from build123d import *

# Parameters (mm, degrees)
BOSS_EXTRUDE1_DEPTH = 3
SKETCH2_W           = 3.5
SKETCH2_H           = 35
CUT_EXTRUDE7_DEPTH  = 3
FILLET5_R           = 1.5


with BuildPart() as part:
    # Sketch1 → Boss-Extrude1 (new body)
    with BuildSketch(Plane.XY):
        Polygon((68.5, 46), (-68.5, 46), (-68.5, 42.5), (-72, 42.5), (-72, 3.5), (-68.5, 3.5), (-68.5, 0), (68.5, 0), (68.5, 3.5), (72, 3.5), (72, 42.5), (68.5, 42.5), align=None)
    extrude(amount=BOSS_EXTRUDE1_DEPTH)

    # Sketch2 → Cut-Extrude7 (cut)
    with BuildSketch(Plane.XY.offset(3)):
        with Locations((-68.25, 23)):
            Rectangle(SKETCH2_W, SKETCH2_H)
        with Locations((68.25, 23)):
            Rectangle(SKETCH2_W, SKETCH2_H)
    extrude(amount=-CUT_EXTRUDE7_DEPTH, mode=Mode.SUBTRACT)

    # Fillet5
    fillet5_edges = [part.edges().sort_by_distance(p)[0] for p in [
        (-70, 5.5, 1.5),
        (-70, 40.5, 1.5),
        (-66.5, 40.5, 1.5),
        (-66.5, 5.5, 1.5),
        (70, 40.5, 1.5),
        (70, 5.5, 1.5),
        (66.5, 5.5, 1.5),
        (66.5, 40.5, 1.5),
    ]]
    fillet(fillet5_edges, radius=FILLET5_R)


solid = part.part
The model under review builds one solid part; all positions refer to its coordinate system, in mm. A direction names the side the tool comes from. Coordinates: 2 decimals unless noted, no trailing zeros. Loops run counter-clockwise (first coordinate to the right, second up) from the corner with the lowest first, then second, coordinate; pieces in that order, holes last. Notation, with made-up numbers: M 10.25,-12.75 L 59.25,-12.75 A33 ccw 59.25,26.25 Z; hole C 27.25,78.25 d5. An arc over 180 degrees is marked long. Put each result on its own line as item: value. Start each with the question number.
Q1. Add section B-B (z = 2.15). Write out the cut boundary in (x, y), and give its area (3 significant figures).
Q2. For faces 5 (the flat face through (-68.5, 44, 1)), 6 (the flat face through (1, 46, 1)), 7 (the flat face through (68.5, 44, 1)), 8 (the flat face through (-70, 3.5, 1)), 9 (the flat face through (66.5, 23, 2)), list the 3-axis set-ups (+Z, -Z, +X, -X, +Y, -Y) from which the entire face can be reached by the end or side of a thin tool; tool diameter is ignored.
Q3. Add section A-A (y = 13). Write out the cut boundary in (x, z), and give its area (3 significant figures).
Q4. Wall thickness on line 1 (X direction, y = 22, z = 0.45); line 2 (X direction, y = 39.5, z = 2.15); line 3 (X direction, y = 43.5, z = 2.3): over which ranges is each line inside the solid? List them lowest first.
Q5. The part is to be moulded in two halves that separate along Y. For faces 1 (the flat face through (70, 42.5, 1)), 2 (the flat face through (-66.5, 23, 2)), 3 (the flat face through (70, 3.5, 1)), 4 (the flat face through (68.5, 2, 1)), say which applies: +Y half, -Y half, draft (parallel to the pull), parting line (faces both ways), or undercut.
Q6. Clearance check with flat-ended pins moving along their axes: pin 1 (1.5 mm diameter, centred on x = -71, z = 1, fed in from +Y); pin 2 (1.5 mm diameter, centred on x = 70.5, z = 1, fed in from -Y); pin 3 (1.5 mm diameter, centred on y = 44, z = 1.5, fed in from +X). State where each tip first meets the part, or that it passes through.
Answers:
1. outline: M -72,3.5 L -68.5,3.5 L -68.5,0 L 68.5,0 L 68.5,3.5 L 72,3.5 L 72,42.5 L 68.5,42.5 L 68.5,46 L -68.5,46 L -68.5,42.5 L -72,42.5 Z; hole M -70,7 A1.5 ccw -68.5,5.5 L -68,5.5 A1.5 ccw -66.5,7 L -66.5,39 A1.5 ccw -68,40.5 L -68.5,40.5 A1.5 ccw -70,39 Z; hole M 66.5,7 A1.5 ccw 68,5.5 L 68.5,5.5 A1.5 ccw 70,7 L 70,39 A1.5 ccw 68.5,40.5 L 68,40.5 A1.5 ccw 66.5,39 Z
1. area: 6,330 mm^2
2. face 5: +Z, -Z, -X, +Y
2. face 6: +Z, -Z, +X, -X, +Y
2. face 7: +Z, -Z, +X, +Y
2. face 8: +Z, -Z, -X, -Y
2. face 9: +Z, -Z
3. outline: M -72,0 L -70,0 L -70,3 L -72,3 Z; M -66.5,0 L 66.5,0 L 66.5,3 L -66.5,3 Z; M 70,0 L 72,0 L 72,3 L 70,3 Z
3. area: 411 mm^2
4. line 1: x = -72 to -70, -66.5 to 66.5, 70 to 72
4. line 2: x = -72 to -69.91, -66.59 to 66.59, 69.91 to 72
4. line 3: x = -68.5 to 68.5
5. face 1: +Y half
5. face 2: undercut
5. face 3: -Y half
5. face 4: draft
6. pin 1: stops at y = 42.5
6. pin 2: stops at y = 3.5
6. pin 3: stops at x = 68.5
